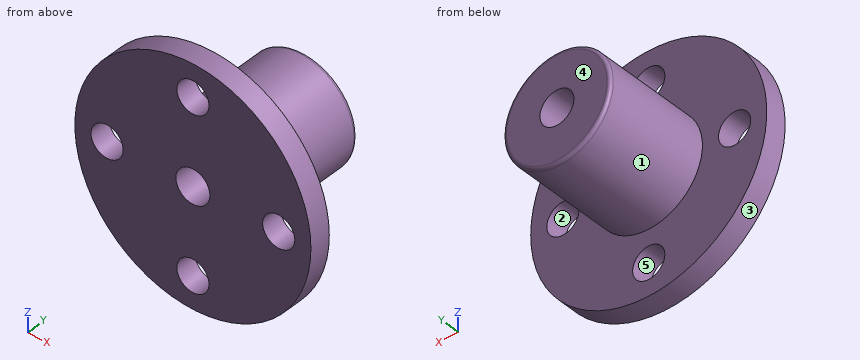
from build123d import *

# Parameters (mm, degrees)
SKETCH1_R           = 11
BOSS_EXTRUDE1_DEPTH = 2
SKETCH2_R           = 5
BOSS_EXTRUDE2_DEPTH = 10
FILLET1_R           = 0.3
SKETCH3_R           = 1.5
CUT_EXTRUDE1_DEPTH  = 10
SKETCH4_R           = 1.585
CUT_EXTRUDE2_DEPTH  = 20


with BuildPart() as part:
    # Sketch1 → Boss-Extrude1 (new body)
    with BuildSketch(Plane(origin=(0, 0, 0), x_dir=(1, 0, 0), z_dir=(0, 1, 0))):
        Circle(SKETCH1_R)
    extrude(amount=BOSS_EXTRUDE1_DEPTH)

    # Sketch2 → Boss-Extrude2 (add)
    with BuildSketch(Plane(origin=(0, 2, 0), x_dir=(1, 0, 0), z_dir=(0, 1, 0))):
        Circle(SKETCH2_R)
    extrude(amount=BOSS_EXTRUDE2_DEPTH)

    # Fillet1
    fillet1_edges = [part.edges().sort_by_distance(p)[0] for p in [
        (-5, 12, 0),
    ]]
    fillet(fillet1_edges, radius=FILLET1_R)

    # Sketch3 → Cut-Extrude1 (cut)
    with BuildSketch(Plane(origin=(0, 2, 0), x_dir=(1, 0, 0), z_dir=(0, 1, 0))):
        with Locations((0, 8)):
            Circle(SKETCH3_R)
        with Locations((8, 0)):
            Circle(SKETCH3_R)
        with Locations((0, -8)):
            Circle(SKETCH3_R)
        with Locations((-8, 0)):
            Circle(SKETCH3_R)
    extrude(amount=-CUT_EXTRUDE1_DEPTH, mode=Mode.SUBTRACT)

    # Sketch4 → Cut-Extrude2 (cut)
    with BuildSketch(Plane(origin=(0, 12, 0), x_dir=(1, 0, 0), z_dir=(0, 1, 0))):
        Circle(SKETCH4_R)
    extrude(amount=-CUT_EXTRUDE2_DEPTH, mode=Mode.SUBTRACT)


solid = part.part
Input: part model. Units: mm. Frame: model coordinates. Face numbers are marked on the shaded views. A direction names the side the tool comes from. Give positions to 0.01 mm unless a question says otherwise; leave off trailing zeros. Order: outer loops, then holes, each group sorted by start corner. A loop starts at its lowest first (then second) coordinate and runs counter-clockwise, first axis right, second up. Notation, with made-up numbers: (20, -20) - (27, -20) arc R22 cw to (27, 16) - close; hole circle Ø3 at (60.25, 55.5). An arc over 180 degrees is marked (long way). Write each question's results on one line, items separated by ' | '.
Item 1: Section C-C (z = 8.5). Return loops of the section in (x, y).
A:
outline: (-6.98, 0) - (-1.41, 0) - (-1.41, 2) - (-6.98, 2) - close; (1.41, 0) - (6.98, 0) - (6.98, 2) - (1.41, 2) - close
Item 2: Draft query along X for the marked faces 3, 4 and 5. Return one class per face: released by +X, released by -X, zero draft, split by the parting line, or undercut.
A:
face 3: split by the parting line | face 4: zero draft | face 5: undercut
Item 3: Section B-B (x = 0). Return loops of the section in (y, z) (3 decimals), and give its area (3 significant figures).
A:
outline: (0, -11) - (2, -11) - (2, -9.5) - (0, -9.5) - close; (0, -6.5) - (2, -6.5) - (2, -5) - (11.7, -5) arc R0.3 ccw to (12, -4.7) - (12, -1.585) - (0, -1.585) - close; (0, 1.585) - (12, 1.585) - (12, 4.7) arc R0.3 ccw to (11.7, 5) - (2, 5) - (2, 6.5) - (0, 6.5) - close; (0, 9.5) - (2, 9.5) - (2, 11) - (0, 11) - close | area: 93.9 mm^2
Item 4: Access query for the marked faces 1 and 2. Directions: +Z, -Z, +X, -X, +Y, -Y. A direction counts if a zero-diameter tool reaches every point of the face in a straight line with its end or side. Return the directions, or none.
A:
face 1: +Y | face 2: +Y, -Y
Item 5: Section A-A (z = 0). Return loops of the section in (x, y) (3 decimals), and give its area (3 significant figures).
A:
outline: (-11, 0) - (-9.5, 0) - (-9.5, 2) - (-11, 2) - close; (-6.5, 0) - (-1.585, 0) - (-1.585, 12) - (-4.7, 12) arc R0.3 ccw to (-5, 11.7) - (-5, 2) - (-6.5, 2) - close; (1.585, 0) - (6.5, 0) - (6.5, 2) - (5, 2) - (5, 11.7) arc R0.3 ccw to (4.7, 12) - (1.585, 12) - close; (9.5, 0) - (11, 0) - (11, 2) - (9.5, 2) - close | area: 93.9 mm^2
Item 6: Material intervals for line 1 along Z through (x, y) = (0, 1.05) (3 decimals); line 2 along Y through (x, z) = (7, -2.5), sorted ascending.
A:
line 1: z = -11 to -9.5, -6.5 to -1.585, 1.585 to 6.5, 9.5 to 11 | line 2: y = 0 to 2
Item 7: Section D-D (x = -7). Return loops of the section in (y, z), and give its area (3 significant figures).
A:
outline: (0, -8.49) - (2, -8.49) - (2, -1.12) - (0, -1.12) - close; (0, 1.12) - (2, 1.12) - (2, 8.49) - (0, 8.49) - close | area: 29.5 mm^2
Item 8: Contact query for flat-ended pins moving along their axis: pin 1 Ø4 at (x, z) = (0, -8) entering from -Y; pin 2 Ø1.5 at (x, y) = (5, 10.5) entering from +Z; pin 3 Ø6 at (x, y) = (-6, 6) entering from +Z; pin 4 Ø1 at (y, z) = (6.5, -4.5) entering from -X. Output: stop coordinate, or through.
A:
pin 1: stops at y = 0 | pin 2: stops at z = 2.63 | pin 3: stops at z = 4 | pin 4: stops at x = -3
